Geometry check sheet. Reference: the model listing, model coordinates, mm. A direction names the side the tool comes from. Round coordinates to 2 decimals unless told otherwise and drop trailing zeros. Write each loop counter-clockwise with the first axis right and the second up, starting at its lowest first coordinate (ties: lowest second). Pieces come first, ordered by that corner, then holes.
Item 1: Draft check along X on faces 1 (the face through (4.583, 0, 1)), 2 (the face through (-2.44, -0.14, -0.54)), 3 (the face through (5.5, -17, -1)). Enter one of: pulls with the +X half, pulls with the -X half, needs draft (parallel to the pull), parting line crosses it, or undercut.
Item 2: Cross-section at C-C (x = 0). Enter the section's corners in (y, z), then the cut area to 3 significant figures.
Item 3: Cross-section at D-D (y = -20). Enter the section's corners in (x, z).
Item 4: Scan lines: probe 1 along X at (y, z) = (20, -1.45); probe 2 along Z at (x, y) = (8, -24.5); probe 3 along X at (y, z) = (18, -0.75). Record each from-to range of solid material in increasing order.
Item 5: Cross-section at A-A (x = 20). Enter the section's corners in (y, z), then the cut area to 3 significant figures.
Item 6: Access from +Z, -Z, +X, -X, +Y, -Y to the whole of each face (thin tool, end or side, straight path). Record for faces 4 (the face through (14, 0, -2)), 5 (the face through (14, 0, 0)), 6 (the face through (16.753, -20.143, -1.137)), 7 (the face through (30, 0, -1)), 8 (the face through (3, -10, 0)).
Item 7: Depth check by flat-ended pin: P1, Ø6, axis at x = 0, z = 0, coming from the +Y side; P2, Ø1.6, axis at y = -19.5, z = -1, coming from the -X side; P3, Ø1.5, axis at x = 8.5, y = -2, coming from the +Z side. Enter the tip coordinate at first touch or a pass-through.
Item 8: Cross-section at B-B (y = 0). Enter the section's corners in (x, z), then the cut area to 3 significant figures.
from build123d import *

# Parameters (mm, degrees)
SKETCH1_W                            = 24.5
SKETCH1_H                            = 2
BOSS_EXTRUDE1_DEPTH                  = 30
SKETCH1_4_R                          = 2.5
BOSS_EXTRUDE2_DEPTH                  = 10
F_6_5_6_5_DIAMETER_HOLE1_D           = 6.5
F_6_5_6_5_DIAMETER_HOLE1_CSINK_D     = 7
F_6_5_6_5_DIAMETER_HOLE1_CSINK_ANGLE = 90
FILLET1_R                            = 5


with BuildPart() as part:
    # Sketch1 → Boss-Extrude1 (new, symmetric)
    with BuildSketch(Plane(origin=(0, 0, 0), x_dir=(1, 0, 0), z_dir=(0, 1, 0))):
        with Locations((17.75, 1)):
            Rectangle(SKETCH1_W, SKETCH1_H)
    extrude(amount=BOSS_EXTRUDE1_DEPTH, both=True)

    # Sketch1_4 → Boss-Extrude2 (add, symmetric)
    with BuildSketch(Plane(origin=(0, 0, 0), x_dir=(1, 0, 0), z_dir=(0, 1, 0))):
        with BuildLine():
            Line((5.5, 0), (5.5, 2))
            Line((5.5, 2), (4.582575695, 2))
            ThreePointArc((4.582575695, 2), (-5, 0), (4.582575695, -2))
            Line((4.582575695, -2), (4.582575695, 0))
            Line((4.582575695, 0), (5.5, 0))
        make_face()
        with Locations(Location((0, 0, 0), (0, 0, 270))):
            Circle(SKETCH1_4_R, mode=Mode.SUBTRACT)
    extrude(amount=BOSS_EXTRUDE2_DEPTH, both=True)

    # 6.5 _6.5_ Diameter Hole1 (through all)
    with Locations(Plane(origin=(0, 0, 0), x_dir=(-1, 0, 0), z_dir=(0, 0, 1))):
        with Locations((-20, 20), (-20, 0), (-20, -20)):
            CounterSinkHole(F_6_5_6_5_DIAMETER_HOLE1_D / 2, F_6_5_6_5_DIAMETER_HOLE1_CSINK_D / 2, counter_sink_angle=F_6_5_6_5_DIAMETER_HOLE1_CSINK_ANGLE)

    # Fillet1
    fillet1_edges = [part.edges().sort_by_distance(p)[0] for p in [
        (30, 30, -1),
        (5.5, 30, -1),
        (30, -30, -1),
        (5.5, -30, -1),
    ]]
    fillet(fillet1_edges, radius=FILLET1_R)


solid = part.part
Resolved:
1. face 1: pulls with the +X half
1. face 2: undercut
1. face 3: pulls with the -X half
2. outline: (-10, -5) - (10, -5) - (10, -2.5) - (-10, -2.5) - close; (-10, 2.5) - (10, 2.5) - (10, 5) - (-10, 5) - close
2. area: 100 mm2
3. outline: (5.5, -2) - (16.75, -2) - (16.75, -0.25) - (16.5, 0) - (5.5, 0) - close; (23.25, -2) - (30, -2) - (30, 0) - (23.5, 0) - (23.25, -0.25) - close
4. probe 1: x = 5.5 to 16.75, 23.25 to 30
4. probe 2: z = -2 to 0
4. probe 3: x = 5.5 to 17.44, 22.56 to 30
5. outline: (-30, -2) - (-23.25, -2) - (-23.25, -0.25) - (-23.5, 0) - (-30, 0) - close; (-16.75, -2) - (-3.25, -2) - (-3.25, -0.25) - (-3.5, 0) - (-16.5, 0) - (-16.75, -0.25) - close; (3.25, -2) - (16.75, -2) - (16.75, -0.25) - (16.5, 0) - (3.5, 0) - (3.25, -0.25) - close; (23.25, -2) - (30, -2) - (30, 0) - (23.5, 0) - (23.25, -0.25) - close
5. area: 80.8 mm2
6. face 4: -Z, +X, +Y, -Y
6. face 5: +Z, +X, +Y, -Y
6. face 6: +Z, -Z
6. face 7: +Z, -Z, +X, +Y, -Y
6. face 8: +Z, -Z, -X, -Y
7. P1: stops at y = 10
7. P2: stops at x = 5.5
7. P3: stops at z = 0
8. outline: (4.58, -2) - (16.75, -2) - (16.75, -0.25) - (16.5, 0) - (4.58, 0) - (4.58, 2) arc R5 ccw (long way) to start; (23.25, -2) - (30, -2) - (30, 0) - (23.5, 0) - (23.25, -0.25) - close; hole circle Ø5 at (0, 0)
8. area: 95.6 mm2
